Geometry: final body of the model. Coordinates: model frame, mm. Face numbers are marked on the shaded views. A direction names the side the tool comes from. Give positions to 0.01 mm unless a question says otherwise; leave off trailing zeros. Loops run counter-clockwise (first coordinate to the right, second up) from the corner with the lowest first, then second, coordinate; pieces in that order, holes last.
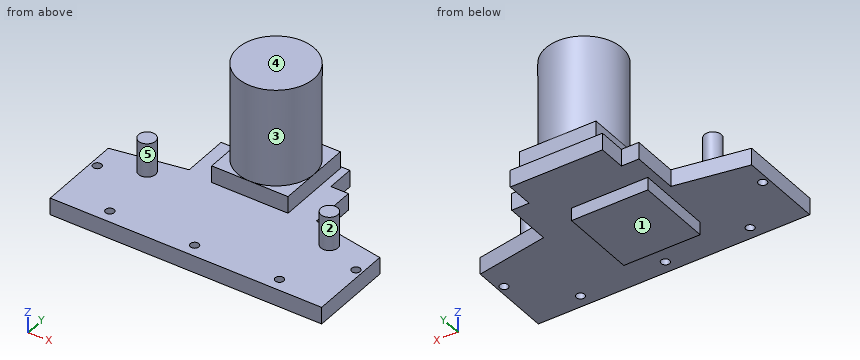
from build123d import *

# Parameters (mm, degrees)
SKETCH1_W           = 30
SKETCH1_H           = 11
SKETCH1_W_2         = 21.75
SKETCH1_H_2         = 6.5
BOSS_EXTRUDE1_DEPTH = 4
SKETCH2_R           = 1
CUT_EXTRUDE1_DEPTH  = 5
SKETCH3_R           = 9
BOSS_EXTRUDE2_DEPTH = 27
SKETCH5_W           = 18
SKETCH5_H           = 18
BOSS_EXTRUDE3_DEPTH = 3
SKETCH6_R           = 2
BOSS_EXTRUDE4_DEPTH = 8
SKETCH7_W           = 18
SKETCH7_H           = 18
BOSS_EXTRUDE5_DEPTH = 4


with BuildPart() as part:
    # Sketch1 → Boss-Extrude1 (new body)
    with BuildSketch(Plane.XY):
        Polygon((32, 0), (32, 20), (15, 23), (-15, 23), (-32, 20), (-32, 0), align=None)
        with Locations((0, 28.5)):
            Rectangle(SKETCH1_W, SKETCH1_H)
        with Locations((0, 37.25)):
            Rectangle(SKETCH1_W_2, SKETCH1_H_2)
    extrude(amount=BOSS_EXTRUDE1_DEPTH)

    # Sketch2 → Cut-Extrude1 (cut)
    with BuildSketch(Plane.XY.offset(4)):
        with Locations((20, 3)):
            Circle(SKETCH2_R)
        with Locations((0, 3)):
            Circle(SKETCH2_R)
        with Locations((-20, 3)):
            Circle(SKETCH2_R)
        with Locations((-30.5, 14)):
            Circle(SKETCH2_R)
        with Locations((30.5, 14)):
            Circle(SKETCH2_R)
    extrude(amount=-CUT_EXTRUDE1_DEPTH, mode=Mode.SUBTRACT)

    # Sketch3 → Boss-Extrude2 (add)
    with BuildSketch(Plane.XY.offset(4)):
        with Locations((0, 31)):
            Circle(SKETCH3_R)
    extrude(amount=BOSS_EXTRUDE2_DEPTH)

    # Sketch5 → Boss-Extrude3 (add)
    with BuildSketch(Plane(origin=(0, 0, 0), x_dir=(-1, 0, 0), z_dir=(0, 0, -1))):
        with Locations((4, 19)):
            Rectangle(SKETCH5_W, SKETCH5_H)
    extrude(amount=BOSS_EXTRUDE3_DEPTH)

    # Sketch6 → Boss-Extrude4 (add)
    with BuildSketch(Plane.XY.offset(4)):
        with Locations((21.5, 18)):
            Circle(SKETCH6_R)
        with Locations((-21.5, 18)):
            Circle(SKETCH6_R)
    extrude(amount=BOSS_EXTRUDE4_DEPTH)

    # Sketch7 → Boss-Extrude5 (add)
    with BuildSketch(Plane.XY.offset(4)):
        with Locations((0, 31)):
            Rectangle(SKETCH7_W, SKETCH7_H)
    extrude(amount=BOSS_EXTRUDE5_DEPTH)


solid = part.part
Item 1: Draft query along X for the marked faces 1, 2 and 3. Return one class per face: +X half, -X half, draft (parallel to the pull), parting line (faces both ways), or undercut.
Values follow:
face 1: draft
face 2: undercut
face 3: parting line
Item 2: Pin query (flat end, axial travel): pin 1 (1 mm diameter, centred on x = 11, y = 4.5, fed in from +Z); pin 2 (12 mm diameter, centred on x = 22, z = 14.5, fed in from -Y); pin 3 (3.5 mm diameter, centred on x = 0.5, z = -2, fed in from +Y); pin 4 (1.2 mm diameter, centred on x = 20, y = 3, fed in from -Z). Return the tip coordinate at first contact, or that it passes through.
Values follow:
pin 1: stops at z = 4
pin 2: stops at y = 16
pin 3: stops at y = 28
pin 4: passes through
Item 3: Ray query, probe 1 along Z at (x, y) = (13.5, 31); probe 2 along X at (y, z) = (23, 6); probe 3 along Y at (x, z) = (21.5, 7). Return the intervals inside material, ascending.
Values follow:
probe 1: z = 0 to 4
probe 2: x = -9 to 9
probe 3: y = 16 to 20
Item 4: Section query C-C on z = 2. Return loops of the section in (x, y) (3 decimals), plus the area to 3 significant figures.
Values follow:
outline: (-32, 0) - (32, 0) - (32, 20) - (15, 23) - (15, 34) - (10.875, 34) - (10.875, 40.5) - (-10.875, 40.5) - (-10.875, 34) - (-15, 34) - (-15, 23) - (-32, 20) - close; hole circle Ø2 at (-30.5, 14); hole circle Ø2 at (-20, 3); hole circle Ø2 at (0, 3); hole circle Ø2 at (20, 3); hole circle Ø2 at (30.5, 14)
area: 1,880 mm2
Item 5: Section query B-B on x = -30.5. Return loops of the section in (y, z), plus the area to 3 significant figures.
Values follow:
outline: (0, 0) - (13, 0) - (13, 4) - (0, 4) - close; (15, 0) - (20.26, 0) - (20.26, 4) - (15, 4) - close
area: 73.1 mm2
Item 6: Section query D-D on y = 18. Return loops of the section in (x, z), plus the area to 3 significant figures.
Values follow:
outline: (-32, 0) - (-13, 0) - (-13, -3) - (5, -3) - (5, 0) - (32, 0) - (32, 4) - (23.5, 4) - (23.5, 12) - (19.5, 12) - (19.5, 4) - (-19.5, 4) - (-19.5, 12) - (-23.5, 12) - (-23.5, 4) - (-32, 4) - close
area: 374 mm2
Item 7: Set-up query: the marked faces 4 and 5. Return all of +Z, -Z, +X, -X, +Y, -Y with unobstructed straight access to the full face (end or side cutting, diameter ignored); none if empty.
Values follow:
face 4: +Z, +X, -X, +Y, -Y
face 5: +Z
Item 8: Section query A-A on y = 3. Return loops of the section in (x, z), plus the area to 3 significant figures.
Values follow:
outline: (-32, 0) - (-21, 0) - (-21, 4) - (-32, 4) - close; (-19, 0) - (-1, 0) - (-1, 4) - (-19, 4) - close; (1, 0) - (19, 0) - (19, 4) - (1, 4) - close; (21, 0) - (32, 0) - (32, 4) - (21, 4) - close
area: 232 mm2
